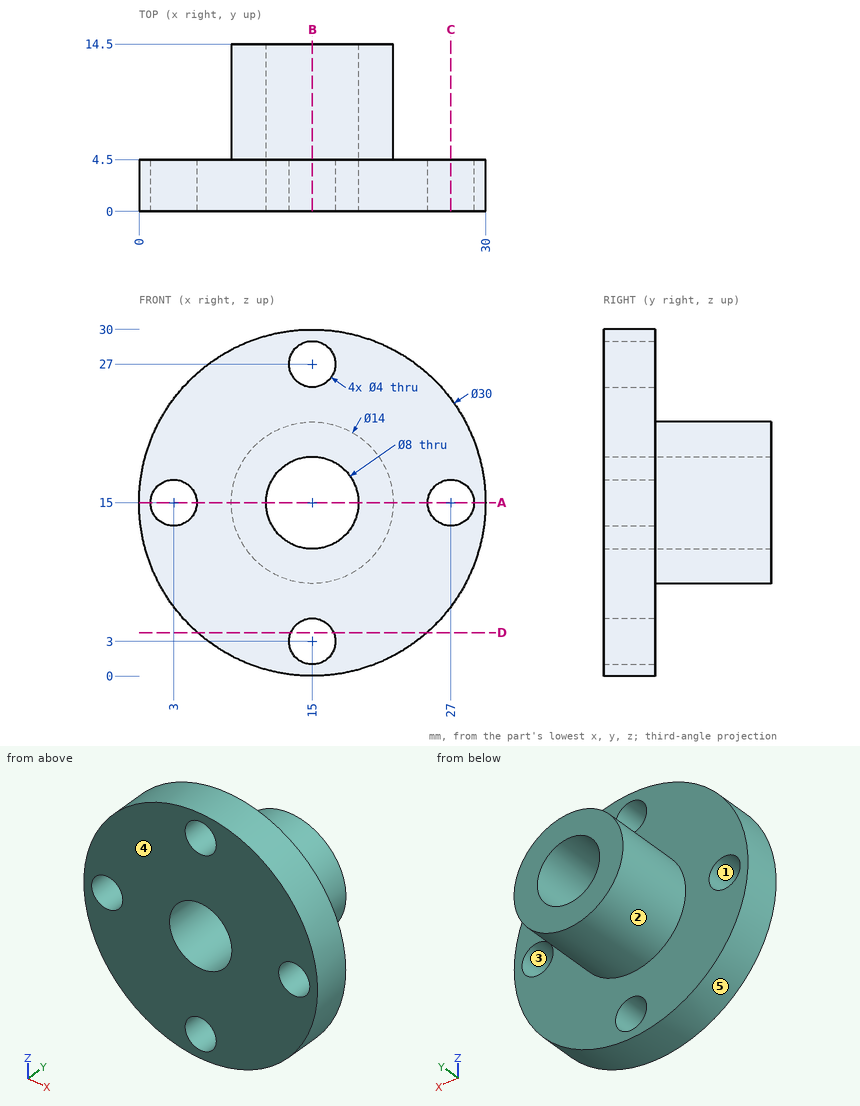
Input: dimensioned drawing with shaded views. Units: mm. Origin: part minimum x, y, z. A direction names the side the tool comes from. Give positions to 0.01 mm unless a question says otherwise; leave off trailing zeros. Write each loop counter-clockwise with the first axis right and the second up, starting at its lowest first coordinate (ties: lowest second). Pieces come first, ordered by that corner, then holes. Notation, with made-up numbers: M 19,42.25 L 64,42.25 A33 ccw 64,77.25 Z; hole C 18,-17 d6. An arc over 180 degrees is marked long. Return JSON: item names as keys, results as strings. Group by question number.
1) Material intervals for line 1 along X through (y, z) = (12, 15); line 2 along X through (y, z) = (3.1, 15); line 3 along X through (y, z) = (2, 14), sorted ascending. Write a range as [from, to].
2) Pull-direction query (Z, two-part tool) for the marked faces 3, 4 and 5; classes: pulls with the +Z half, pulls with the -Z half, needs draft (parallel to the pull), parting line crosses it, or undercut.
3) Cut plane A-A, the plane z = 15. Output: boundary loops of the cut face in (x, y).
4) Set-up query: the marked faces 1 and 2. Return all of +Z, -Z, +X, -X, +Y, -Y with unobstructed straight access to the full face (end or side cutting, diameter ignored); none if empty.
5) Cut plane B-B, the plane x = 15. Output: boundary loops of the cut face in (y, z), plus the area to 3 significant figures.
6) Cut plane D-D, the plane z = 3.75. Output: boundary loops of the cut face in (x, y).
7) Pin query (flat end, axial travel): P1, Ø3, axis at x = 15, z = 3, coming from the -Y side; P2, Ø2, axis at x = 12, z = 4.5, coming from the +Y side; P3, Ø5, axis at y = 8.5, z = 14.5, coming from the +X side; P4, Ø3, axis at y = 10.5, z = 10.5, coming from the -X side. Return the tip coordinate at first contact, or that it passes through.
8) Cut plane C-C, the plane x = 27. Output: boundary loops of the cut face in (y, z).
Recorded:
{
 "1": {"line 1": "x = [8, 11], [19, 22]", "line 2": "x = [0, 1], [5, 11], [19, 25], [29, 30]", "line 3": "x = [0.03, 1.27], [4.73, 11.13], [18.87, 25.27], [28.73, 29.97]"},
 "2": {"face 3": "undercut", "face 4": "needs draft", "face 5": "parting line crosses it"},
 "3": {"outline": "M 0,0 L 1,0 L 1,4.5 L 0,4.5 Z; M 5,0 L 11,0 L 11,14.5 L 8,14.5 L 8,4.5 L 5,4.5 Z; M 19,0 L 25,0 L 25,4.5 L 22,4.5 L 22,14.5 L 19,14.5 Z; M 29,0 L 30,0 L 30,4.5 L 29,4.5 Z"},
 "4": {"face 1": "+Y, -Y", "face 2": "+Y"},
 "5": {"outline": "M 0,0 L 4.5,0 L 4.5,1 L 0,1 Z; M 0,5 L 4.5,5 L 4.5,8 L 14.5,8 L 14.5,11 L 0,11 Z; M 0,19 L 14.5,19 L 14.5,22 L 4.5,22 L 4.5,25 L 0,25 Z; M 0,29 L 4.5,29 L 4.5,30 L 0,30 Z", "area": "123 mm²"},
 "6": {"outline": "M 5.08,0 L 13.15,0 L 13.15,4.5 L 5.08,4.5 Z; M 16.85,0 L 24.92,0 L 24.92,4.5 L 16.85,4.5 Z"},
 "7": {"P1": "passes through", "P2": "stops at y = 4.5", "P3": "stops at x = 22", "P4": "stops at x = 8.68"},
 "8": {"outline": "M 0,6 L 4.5,6 L 4.5,13 L 0,13 Z; M 0,17 L 4.5,17 L 4.5,24 L 0,24 Z"}
}
